CAD build for the part. Positions are in the model's coordinates, mm. A direction names the side the tool comes from. Round coordinates to 2 decimals unless told otherwise and drop trailing zeros. Loops run counter-clockwise (first coordinate to the right, second up) from the corner with the lowest first, then second, coordinate; pieces in that order, holes last. Notation, with made-up numbers: M 42.25,-10.75 L 49.25,-10.75 A24 cw 49.25,23.25 Z; hole C -37.5,-35 d7. An arc over 180 degrees is marked long. Put each result on its own line as item: value. Start each with the question number.
Autodesk Inventor part; units mm, degrees
ref_plane "YZ Plane" through (0, 0, 0) normal (1, 0, 0) x (0, 1, 0)
ref_plane "XZ Plane" through (0, 0, 0) normal (0, 1, 0) x (-1, 0, 0)
ref_plane "XY Plane" through (0, 0, 0) normal (0, 0, 1) x (1, 0, 0)
sketch "Sketch1" plane through (0, 0, 0) normal (0, 1, 0) x (-1, 0, 0)
  circle A0 centre (0, 0) radius 30
  circle A1 centre (0, 0) radius 32.5
  circle A2 centre (0, 0) radius 35
  dimension "d0" = 60
  dimension "d1" = 65
  dimension "d2" = 70
extrude "Extrusion1" add sketch "Sketch1" along normal blind 46 contours A1
extrude "Extrusion2" add sketch "Sketch1" along normal blind 44 and the other way blind 2 contours A2
properties part number "electronicschamber" material "ABS Plastic"
(1) Cut at C-C on y = 5. List the corners of the cut face in (x, z).
(2) Mould opens along Z. For faces 3 (the cylindrical face through (-31, 44.99, -9.76)), 4 (the flat face through (-23.2, 44, -23.2)), 5 (the cylindrical face through (-31, -0.99, 9.76)) say: +Z half, -Z half, draft (parallel to the pull), parting line (faces both ways), or undercut.
(3) Drill centre lines: line 1 along X through (y, z) = (10, 1); line 2 along Z through (x, y) = (0, -1); line 3 along Z through (x, y) = (26, 25). Where is each one in solid material? Low to high.
(4) Flat gauge pins, fed straight in: pin 1 Ø1.5 at (x, y) = (27.5, 7) entering from +Z; pin 2 Ø4 at (y, z) = (5, -18) entering from -X; pin 3 Ø5 at (x, z) = (18.5, 18) entering from +Y; pin 4 Ø8 at (x, y) = (-15.5, 16) entering from -Z. Where does each tip first touch, or does it go through?
(5) Cut at B-B on x = 0. List the corners of the cut face in (y, z).
(6) Cut at A-A on z = 0. List the corners of the cut face in (x, y), and give its area (3 significant figures).
(7) Tool access for faces 1 (the flat face through (-9, 0, -29)), 2 (the cylindrical face through (29.97, 22.68, -1.32)): list every direction of +Z, -Z, +X, -X, +Y, -Y with a clear straight run to the whole face (end or side of a thin tool).
Taken from the geometry:
1. outline: C 0,0 d70; hole C 0,0 d60
2. face 3: parting line
2. face 4: draft
2. face 5: undercut
3. line 1: -34.99 to -29.98, 29.98 to 34.99
3. line 2: -35 to -32.5, 32.5 to 35
3. line 3: -23.43 to -14.97, 14.97 to 23.43
4. pin 1: z = 22.57
4. pin 2: x = -31.13
4. pin 3: through
4. pin 4: z = -33.06
5. outline: M -2,-35 L 44,-35 L 44,-32.5 L 46,-32.5 L 46,-30 L 0,-30 L 0,-32.5 L -2,-32.5 Z; M -2,32.5 L 0,32.5 L 0,30 L 46,30 L 46,32.5 L 44,32.5 L 44,35 L -2,35 Z
6. outline: M -35,-2 L -32.5,-2 L -32.5,0 L -30,0 L -30,46 L -32.5,46 L -32.5,44 L -35,44 Z; M 30,0 L 32.5,0 L 32.5,-2 L 35,-2 L 35,44 L 32.5,44 L 32.5,46 L 30,46 Z
6. area: 460 mm2
7. face 1: -Y
7. face 2: +Y, -Y
